```python
from build123d import *

# Parameters (mm, degrees)
SKETCH1_W           = 90.8
SKETCH1_H           = 31
BOSS_EXTRUDE1_DEPTH = 3
SKETCH2_R           = 0.95
CUT_EXTRUDE1_DEPTH  = 3
SKETCH3_R           = 1.9
CUT_EXTRUDE2_DEPTH  = 2
SKETCH4_W           = 54
SKETCH4_H           = 7
BOSS_EXTRUDE2_DEPTH = 5
SKETCH5_R           = 3.9
CUT_EXTRUDE3_DEPTH  = 54
FILLET1_R           = 7


with BuildPart() as part:
    # Sketch1 → Boss-Extrude1 (new body)
    with BuildSketch(Plane(origin=(0, 0, 0), x_dir=(1, 0, 0), z_dir=(0, 1, 0))):
        Rectangle(SKETCH1_W, SKETCH1_H)
    extrude(amount=BOSS_EXTRUDE1_DEPTH)

    # Sketch2 → Cut-Extrude1 (cut)
    with BuildSketch(Plane(origin=(0, 3, 0), x_dir=(1, 0, 0), z_dir=(0, 1, 0))):
        with Locations(Location((-34.4, 9.5, 0), (0, 0, 270))):
            Circle(SKETCH2_R)
        with Locations(Location((34.4, 9.5, 0), (0, 0, 270))):
            Circle(SKETCH2_R)
        with Locations(Location((-34.4, -9.5, 0), (0, 0, 270))):
            Circle(SKETCH2_R)
        with Locations(Location((34.4, -9.5, 0), (0, 0, 270))):
            Circle(SKETCH2_R)
    extrude(amount=-CUT_EXTRUDE1_DEPTH, mode=Mode.SUBTRACT)

    # Sketch3 → Cut-Extrude2 (cut)
    with BuildSketch(Plane(origin=(0, 3, 0), x_dir=(1, 0, 0), z_dir=(0, 1, 0))):
        with Locations(Location((-34.4, 9.5, 0), (0, 0, 270))):
            Circle(SKETCH3_R)
        with Locations(Location((-34.4, -9.5, 0), (0, 0, 270))):
            Circle(SKETCH3_R)
        with Locations(Location((34.4, 9.5, 0), (0, 0, 270))):
            Circle(SKETCH3_R)
        with Locations(Location((34.4, -9.5, 0), (0, 0, 270))):
            Circle(SKETCH3_R)
    extrude(amount=-CUT_EXTRUDE2_DEPTH, mode=Mode.SUBTRACT)

    # Sketch4 → Boss-Extrude2 (add)
    with BuildSketch(Plane.XZ):
        Rectangle(SKETCH4_W, SKETCH4_H)
    extrude(amount=BOSS_EXTRUDE2_DEPTH)

    # Sketch5 → Cut-Extrude3 (cut)
    with BuildSketch(Plane(origin=(27, 0, 0), x_dir=(0, 0, -1), z_dir=(1, 0, 0))):
        with Locations((0, -6.130658567)):
            Circle(SKETCH5_R)
    extrude(amount=-CUT_EXTRUDE3_DEPTH, mode=Mode.SUBTRACT)

    # Fillet1
    # the kernel refuses this fillet: 7 mm, written as the material it takes off along each edge
    with BuildSketch(Plane(origin=(59.761406616, 3, 15.5), x_dir=(0, 0, -1), z_dir=(-1, 0, 0))) as fillet1_piece_1:
        with BuildLine():
            CenterArc((5.744562647, 7), FILLET1_R, 214.849904579, 55.150095421)
            Line((0, 3), (-0.114891253, 2.92))
            ThreePointArc((-0.114891253, 2.92), (-0.14, 1.5), (-0.14, 0))
            Line((-0.14, 0), (0, -0.14))
            Line((0, -0.14), (5.744562647, -0.14))
            Line((5.744562647, -0.14), (5.744562647, 0))
        make_face()
    extrude(amount=119.522813233, mode=Mode.SUBTRACT)
    with BuildSketch(Plane(origin=(-59.761406616, 3, -15.5), x_dir=(0, -1, 0), z_dir=(1, 0, 0))) as fillet1_piece_2:
        with BuildLine():
            CenterArc((7, -5.744562647), FILLET1_R, 124.849904579, 55.150095421)
            Line((0, -5.744562647), (-0.14, -5.744562647))
            Line((-0.14, -5.744562647), (-0.14, 0))
            Line((-0.14, 0), (0, 0.14))
            ThreePointArc((0, 0.14), (1.5, 0.14), (2.92, 0.114891253))
            Line((2.92, 0.114891253), (3, 0))
        make_face()
    extrude(amount=119.522813233, mode=Mode.SUBTRACT)


solid = part.part
```
Part model, mm, in its own coordinate system. A direction names the side the tool comes from. Round coordinates to 2 decimals unless told otherwise and drop trailing zeros. Write each loop counter-clockwise with the first axis right and the second up, starting at its lowest first coordinate (ties: lowest second). Pieces come first, ordered by that corner, then holes. Notation, with made-up numbers: (48.5, 11.25) -> (99.5, 11.25) arc R21 cw to (99.5, 39.25) -> close; hole circle Ø5 at (82, 38.25). An arc over 180 degrees is marked (long way). Return JSON: item names as keys, results as strings. Group by question number.
Q1. Probe L1, parallel to X at y = 1.6, z = 9.5; L2, parallel to X at y = 0.7, z = 9.5; L3, parallel to Z at x = 34.4, y = 1.9. List the from-to ranges inside material, lowest first. Write a range as [from, to].
Q2. Saw through at B-B on y = 2. Write the cut outline in (x, z).
Q3. Saw through at D-D on x = 25.5. Write the cut outline in (y, z).
Q4. Mould opens along Z. For faces 5 (the flat face through (27, -2, 0)), 6 (the cylindrical face through (0.38, -2.23, -0.06)), 7 (the cylindrical face through (-0.64, 2.18, -13.04)) say: pulls with the +Z half, pulls with the -Z half, needs draft (parallel to the pull), parting line crosses it, or undercut.
Q5. Saw through at A-A on x = -34.4. Write the cut outline in (y, z).
Q6. Pin check, flat tips, straight feed: pin 1 (1.1 mm diameter, centred on x = 35, z = 9, fed in from +Y); pin 2 (1.3 mm diameter, centred on y = -1, z = 1.5, fed in from -X); pin 3 (4.5 mm diameter, centred on x = 34.4, z = 9.5, fed in from +Y); pin 4 (1.3 mm diameter, centred on y = -3, z = 0, fed in from +X). Stop position of each tip, or through.
Q7. Which spindle directions (+Z, -Z, +X, -X, +Y, -Y) get a long thin tool onto all of the face, cutting with end or side? Do faces 1 (the cylindrical face through (34.971, 2.014, -7.688)), 2 (the flat face through (0, -2, -3.5)), 3 (the flat face through (-27, -2, 0)), 4 (the cylindrical face through (34.44, 0.51, -10.45)). Say none if no direction does.
Q8. Saw through at C-C on z = 6. Write the cut outline in (x, y), plus the area to 3 significant figures.
Answer:
{
 "1": {"L1": "[-45.4, -36.3], [-32.5, 32.5], [36.3, 45.4]", "L2": "[-45.4, -35.35], [-33.45, 33.45], [35.35, 45.4]", "L3": "[-13.52, -11.4], [-7.6, 7.6], [11.4, 13.52]"},
 "2": {"outline": "(-45.4, -13.36) -> (45.4, -13.36) -> (45.4, 13.36) -> (-45.4, 13.36) -> close; hole circle Ø3.8 at (-34.4, -9.5); hole circle Ø3.8 at (-34.4, 9.5); hole circle Ø3.8 at (34.4, -9.5); hole circle Ø3.8 at (34.4, 9.5)"},
 "3": {"outline": "(-4.41, -3.5) -> (0, -3.5) -> (0, -15.5) arc R7 ccw to (3, -9.76) -> (3, 9.76) arc R7 ccw to (0, 15.5) -> (0, 3.5) -> (-4.41, 3.5) arc R3.9 cw to start"},
 "4": {"face 5": "needs draft", "face 6": "undercut", "face 7": "pulls with the -Z half"},
 "5": {"outline": "(0, -15.5) arc R7 ccw to (2.8, -11.4) -> (1, -11.4) -> (1, -10.45) -> (0, -10.45) -> close; (0, -8.55) -> (1, -8.55) -> (1, -7.6) -> (3, -7.6) -> (3, 7.6) -> (1, 7.6) -> (1, 8.55) -> (0, 8.55) -> close; (0, 10.45) -> (1, 10.45) -> (1, 11.4) -> (2.8, 11.4) arc R7 ccw to (0, 15.5) -> close"},
 "6": {"pin 1": "y = 1", "pin 2": "x = -27", "pin 3": "y = 3", "pin 4": "through"},
 "7": {"face 1": "+Y", "face 2": "-Z, +X, -X, -Y", "face 3": "+Z, -Z, -X, -Y", "face 4": "+Y, -Y"},
 "8": {"outline": "(-45.4, 0) -> (45.4, 0) -> (45.4, 3) -> (-45.4, 3) -> close", "area": "272 mm2"}
}
